Check sheet for the modelled part. Datum: model origin and axes. Units: mm. A direction names the side the tool comes from. Coordinates: 2 decimals unless noted, no trailing zeros. Write each loop counter-clockwise with the first axis right and the second up, starting at its lowest first coordinate (ties: lowest second). Pieces come first, ordered by that corner, then holes. Notation, with made-up numbers: (62.25, -13) - (90.25, -13) arc R12 cw to (90.25, 0) - close; hole circle Ø1 at (36, 65.25). An arc over 180 degrees is marked (long way). Write each question's results on one line, items separated by ' | '.
from build123d import *

# Parameters (mm, degrees)
F0_R     = 10
F0_R_2   = 3.75
F0_R_3   = 2.25
F1_DEPTH = 2
F2_DEPTH = 4.75
F3_DEPTH = 2.5


with BuildPart() as f1:
    # F0 (on Top) → F1 (new body)
    with BuildSketch(Plane.XY):
        Circle(F0_R)
        Circle(F0_R_2, mode=Mode.SUBTRACT)
        Circle(F0_R_2)
        Circle(F0_R_3, mode=Mode.SUBTRACT)
    extrude(amount=F1_DEPTH)

    # F0 (on Top) → F2 (join)
    with BuildSketch(Plane.XY):
        Circle(F0_R_3)
    extrude(amount=F2_DEPTH)

    # F0 (on Top) → F3 (join)
    with BuildSketch(Plane.XY):
        Circle(F0_R_2)
        Circle(F0_R_3, mode=Mode.SUBTRACT)
    extrude(amount=F3_DEPTH)


solid = f1.part
1. Sectioned sample at A-A (x = 0). Record the cut outline in (y, z).
Values follow:
outline: (-10, 0) - (10, 0) - (10, 2) - (3.75, 2) - (3.75, 2.5) - (2.25, 2.5) - (2.25, 4.75) - (-2.25, 4.75) - (-2.25, 2.5) - (-3.75, 2.5) - (-3.75, 2) - (-10, 2) - close
2. Sectioned sample at B-B (y = -0.75). Record the cut outline in (x, z), then the cut area to 3 significant figures.
Values follow:
outline: (-9.97, 0) - (9.97, 0) - (9.97, 2) - (3.67, 2) - (3.67, 2.5) - (2.12, 2.5) - (2.12, 4.75) - (-2.12, 4.75) - (-2.12, 2.5) - (-3.67, 2.5) - (-3.67, 2) - (-9.97, 2) - close | area: 53.1 mm^2
3. Material ranges on L1, parallel to Z at x = -5, y = -2; L2, parallel to Z at x = -3.25, y = 0.5; L3, parallel to X at y = -2.75, z = 2.05, recorded low to high. Write a range as [from, to].
Values follow:
L1: z = [0, 2] | L2: z = [0, 2.5] | L3: x = [-2.55, 2.55]
4. Sectioned sample at D-D (z = 3.5). Record the cut outline in (x, y), then the cut area to 3 significant figures.
Values follow:
outline: circle Ø4.5 at (0, 0) | area: 15.9 mm^2
5. Access from +Z, -Z, +X, -X, +Y, -Y to the whole of each face (thin tool, end or side, straight path). Record for faces 1 (the cylindrical face through (-3.746, 0.165, 2.246)), 2 (the flat face through (0, 0, 0)).
Values follow:
face 1: +Z | face 2: -Z, +X, -X, +Y, -Y
6. Go/stop test with flat-tipped pins: pin 1 (1.5 mm diameter, centred on y = -2, z = 1, fed in from -X); pin 2 (3 mm diameter, centred on x = -7, y = -3, fed in from +Z); pin 3 (1 mm diameter, centred on x = -2.5, y = -2, fed in from +Z). Record where each tip stops, or that it passes through.
Values follow:
pin 1: stops at x = -9.92 | pin 2: stops at z = 2 | pin 3: stops at z = 2.5
7. Sectioned sample at C-C (z = 1.1). Record the cut outline in (x, y).
Values follow:
outline: circle Ø20 at (0, 0)
